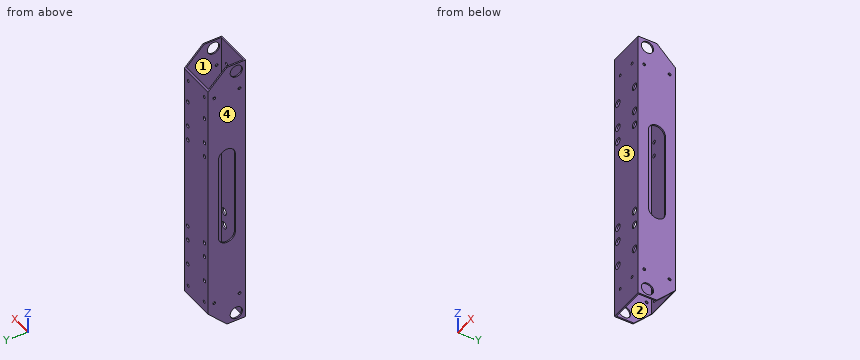
from build123d import *

# Parameters (mm, degrees)
SKETCH_1_W          = 40
SKETCH_1_H          = 40
SKETCH_1_W_2        = 37
SKETCH_1_H_2        = 37
EXTRUDE_1_DEPTH     = 148.75
SKETCH_2_R          = 6.5
CUT_EXTRUDE_1_DEPTH = 45
SKETCH_3_R          = 2.025
CUT_EXTRUDE_2_DEPTH = 50
SKETCH_4_R          = 3.75
CUT_EXTRUDE_3_DEPTH = 3
SKETCH_5_R          = 2.025
CUT_EXTRUDE_4_DEPTH = 60
SKETCH_6_R          = 3.75
CUT_EXTRUDE_5_DEPTH = 3
SKETCH_7_R          = 1.55
CUT_EXTRUDE_6_DEPTH = 55
SKETCH_8_R          = 1.525
CUT_EXTRUDE_7_DEPTH = 20
SKETCH_9_R          = 1.525
CUT_EXTRUDE_8_DEPTH = 3


with BuildPart() as part:
    # 草图1 → 凸台-拉伸1 (new, symmetric)
    with BuildSketch(Plane.XY):
        Rectangle(SKETCH_1_W, SKETCH_1_H)
        Rectangle(SKETCH_1_W_2, SKETCH_1_H_2, mode=Mode.SUBTRACT)
    extrude(amount=EXTRUDE_1_DEPTH, both=True)

    # 草图2 → 切除-拉伸1 (cut)
    with BuildSketch(Plane(origin=(20, 0, 0), x_dir=(0, 0, -1), z_dir=(1, 0, 0))):
        with Locations(Location((-140, -10, 0), (0, 0, 90))):
            Circle(SKETCH_2_R)
        with Locations(Location((140, -10, 0), (0, 0, 90))):
            Circle(SKETCH_2_R)
        Polygon((-148.75, 0), (-128.75, 20), (-148.75, 20), align=None)
        with BuildLine():
            Line((-45, 9), (45, 9))
            ThreePointArc((45, 9), (54, 0), (45, -9))
            Line((45, -9), (-45, -9))
            ThreePointArc((-45, -9), (-54, 0), (-45, 9))
        make_face()
        Polygon((128.75, 20), (148.75, 20), (148.75, 0), align=None)
    extrude(amount=-CUT_EXTRUDE_1_DEPTH, mode=Mode.SUBTRACT)

    # 草图3 → 切除-拉伸2 (cut)
    with BuildSketch(Plane(origin=(0, 20, 0), x_dir=(1, 0, 0), z_dir=(0, 1, 0))):
        with Locations(Location((-14, 50, 0), (0, 0, 270))):
            Circle(SKETCH_3_R)
        with Locations(Location((14, 50, 0), (0, 0, 270))):
            Circle(SKETCH_3_R)
        with Locations(Location((14, -50, 0), (0, 0, 270))):
            Circle(SKETCH_3_R)
        with Locations(Location((-14, -50, 0), (0, 0, 270))):
            Circle(SKETCH_3_R)
    extrude(amount=-CUT_EXTRUDE_2_DEPTH, mode=Mode.SUBTRACT)

    # 草图4 → 切除-拉伸3 (cut)
    with BuildSketch(Plane.XZ.offset(20)):
        with Locations(Location((-14, 50, 0), (0, 0, 270))):
            Circle(SKETCH_4_R)
        with Locations(Location((14, 50, 0), (0, 0, 270))):
            Circle(SKETCH_4_R)
        with Locations(Location((-14, -50, 0), (0, 0, 270))):
            Circle(SKETCH_4_R)
        with Locations(Location((14, -50, 0), (0, 0, 270))):
            Circle(SKETCH_4_R)
    extrude(amount=-CUT_EXTRUDE_3_DEPTH, mode=Mode.SUBTRACT)

    # 草图5 → 切除-拉伸4 (cut)
    with BuildSketch(Plane(origin=(0, 20, 0), x_dir=(1, 0, 0), z_dir=(0, 1, 0))):
        with Locations(Location((-14, 94, 0), (0, 0, 270))):
            Circle(SKETCH_5_R)
        with Locations(Location((14, 94, 0), (0, 0, 270))):
            Circle(SKETCH_5_R)
        with Locations(Location((14, 66, 0), (0, 0, 270))):
            Circle(SKETCH_5_R)
        with Locations(Location((-14, 66, 0), (0, 0, 270))):
            Circle(SKETCH_5_R)
    cut_extrude_4 = extrude(amount=-CUT_EXTRUDE_4_DEPTH, mode=Mode.SUBTRACT)

    # 草图6 → 切除-拉伸5 (cut)
    with BuildSketch(Plane.XZ.offset(20)):
        with Locations(Location((-14, -66, 0), (0, 0, 270))):
            Circle(SKETCH_6_R)
        with Locations(Location((14, -66, 0), (0, 0, 270))):
            Circle(SKETCH_6_R)
        with Locations(Location((-14, -94, 0), (0, 0, 270))):
            Circle(SKETCH_6_R)
        with Locations(Location((14, -94, 0), (0, 0, 270))):
            Circle(SKETCH_6_R)
    cut_extrude_5 = extrude(amount=-CUT_EXTRUDE_5_DEPTH, mode=Mode.SUBTRACT)

    # 镜向1: 切除-拉伸4, 切除-拉伸5 across plane
    add(cut_extrude_4.mirror(Plane.XY), mode=Mode.SUBTRACT)
    add(cut_extrude_5.mirror(Plane.XY), mode=Mode.SUBTRACT)

    # 草图7 → 切除-拉伸6 (cut)
    with BuildSketch(Plane.ZY.offset(20)):
        with Locations(Location((-118.75, 13.45, 0), (0, 0, 270))):
            Circle(SKETCH_7_R)
        with Locations(Location((-118.75, -13.45, 0), (0, 0, 270))):
            Circle(SKETCH_7_R)
    cut_extrude_6 = extrude(amount=-CUT_EXTRUDE_6_DEPTH, mode=Mode.SUBTRACT)

    # 草图8 → 切除-拉伸7 (cut)
    with BuildSketch(Plane(origin=(0, 20, 0), x_dir=(1, 0, 0), z_dir=(0, 1, 0))):
        with Locations(Location((-13.45, 118.75, 0), (0, 0, 270))):
            Circle(SKETCH_8_R)
        with Locations(Location((13.45, 118.75, 0), (0, 0, 270))):
            Circle(SKETCH_8_R)
    cut_extrude_7 = extrude(amount=-CUT_EXTRUDE_7_DEPTH, mode=Mode.SUBTRACT)

    # 镜向2: 切除-拉伸6, 切除-拉伸7 across plane
    add(cut_extrude_6.mirror(Plane.XY), mode=Mode.SUBTRACT)
    add(cut_extrude_7.mirror(Plane.XY), mode=Mode.SUBTRACT)

    # 草图9 → 切除-拉伸8 (cut)
    with BuildSketch(Plane.XZ.offset(20)):
        with Locations((-10, -123.75)):
            Circle(SKETCH_9_R)
        with Locations((10, -123.75)):
            Circle(SKETCH_9_R)
        with Locations(Location((10, 123.75, 0), (0, 0, 90))):
            Circle(SKETCH_9_R)
        with Locations(Location((-10, 123.75, 0), (0, 0, 90))):
            Circle(SKETCH_9_R)
    extrude(amount=-CUT_EXTRUDE_8_DEPTH, mode=Mode.SUBTRACT)


solid = part.part
Design review of the part built by this model. Coordinates are the model's own, in mm. Face numbers are marked on the shaded views. Give positions to 0.01 mm unless a question says otherwise; leave off trailing zeros. Loops run counter-clockwise (first coordinate to the right, second up) from the corner with the lowest first, then second, coordinate; pieces in that order, holes last. Notation, with made-up numbers: M 68.5,34 L 125.5,34 A10 cw 125.5,41 Z; hole C -36,32 d5. An arc over 180 degrees is marked long. One line per question, with ' | ' between items. Start each with the question number.
1. Add section A-A (z = -140). Write out the cut boundary in (x, y), plus the area to 3 significant figures.
2. The part is to be moulded in two halves that separate along X. For the marked faces 1, 2, 3 and 4, say which applies: released by +X, released by -X, zero draft, split by the parting line, or undercut.
3. Insertion check: P1, Ø2.5, axis at x = 14, z = 94, coming from the -Y side. The pin has a flat end and moves straight along its axis. Give the tip position at first contact, or say it passes through.
4. Add section B-B (x = -2). Write out the cut boundary in (y, z), plus the area to 3 significant figures.
5. Add section C-C (z = -31.5). Write out the cut boundary in (x, y), plus the area to 3 significant figures.
6. Add section D-D (y = 4.5). Write out the cut boundary in (x, z).
7. To check wall thickness, follow L1, parallel to X at y = 18.9, z = 94 (3 decimals); L2, parallel to X at y = -19.6, z = 50; L3, parallel to Y at x = -19.65, z = -118.75. State the ranges of each line that lie inside material, in increasing order.
Worked out:
1) outline: M -20,-20 L 20,-20 L 20,-16.5 L 18.5,-16.5 L 18.5,-18.5 L -18.5,-18.5 L -18.5,-16.5 L -20,-16.5 Z; M -20,-3.5 L -18.5,-3.5 L -18.5,8.75 L -20,8.75 Z; M 18.5,-3.5 L 20,-3.5 L 20,8.75 L 18.5,8.75 Z | area: 103 mm²
2) face 1: undercut | face 2: undercut | face 3: zero draft | face 4: released by -X
3) P1: passes through
4) outline: M -20,-148.75 L -18.5,-148.75 L -18.5,148.75 L -20,148.75 Z; M 18.5,-130.25 L 20,-128.75 L 20,128.75 L 18.5,130.25 Z | area: 835 mm²
5) outline: M -20,-20 L 20,-20 L 20,-9 L 18.5,-9 L 18.5,-18.5 L -18.5,-18.5 L -18.5,-9 L -20,-9 Z; M -20,9 L -18.5,9 L -18.5,18.5 L 18.5,18.5 L 18.5,9 L 20,9 L 20,20 L -20,20 Z | area: 177 mm²
6) outline: M -20,-144.25 L -18.5,-144.25 L -18.5,-52.79 L -20,-52.79 Z; M -20,52.79 L -18.5,52.79 L -18.5,144.25 L -20,144.25 Z; M 18.5,-144.25 L 20,-144.25 L 20,-52.79 L 18.5,-52.79 Z; M 18.5,52.79 L 20,52.79 L 20,144.25 L 18.5,144.25 Z
7) L1: x = -20 to -16.025, -11.975 to 11.975, 16.025 to 20 | L2: x = -20 to -17.75, -10.25 to 10.25, 17.75 to 20 | L3: y = -20 to -15, -11.9 to 11.9, 15 to 20
